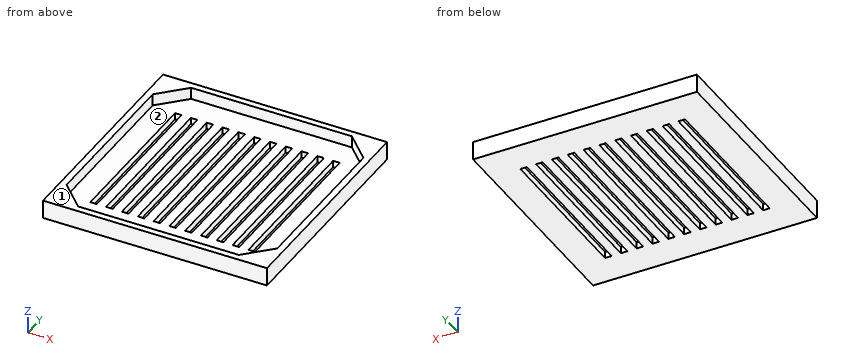
```python
from build123d import *

# Parameters (mm, degrees)
F0_W     = 85
F0_H     = 85
F1_DEPTH = 7
F3_DEPTH = 4.5
F4_W     = 2.5
F4_H     = 60
F5_DEPTH = 25


with BuildPart() as f1:
    # F0 (on Top) → F1 (new body)
    with BuildSketch(Plane.XY):
        Rectangle(F0_W, F0_H)
    extrude(amount=F1_DEPTH)

    # F2 (on face) → F3 (cut)
    with BuildSketch(Plane.XY.offset(7)):
        Polygon((30.5, 40), (-30.5, 40), (-40, 30.5), (-40, -30.5), (-30.5, -40), (30.5, -40), (40, -30.5), (40, 30.5), align=None)
    extrude(amount=-F3_DEPTH, mode=Mode.SUBTRACT)

    # F4 (on face) → F5 (cut)
    with BuildSketch(Plane.XY.offset(7)):
        with Locations((-30.000278, 0)):
            Rectangle(F4_W, F4_H)
        with Locations((-24.000278, 0)):
            Rectangle(F4_W, F4_H)
        with Locations((-18.000278, 0)):
            Rectangle(F4_W, F4_H)
        with Locations((-12.000278, 0)):
            Rectangle(F4_W, F4_H)
        with Locations((-6.000278, 0)):
            Rectangle(F4_W, F4_H)
        with Locations((-0.000278, 0)):
            Rectangle(F4_W, F4_H)
        with Locations((5.999722, 0)):
            Rectangle(F4_W, F4_H)
        with Locations((11.999722, 0)):
            Rectangle(F4_W, F4_H)
        with Locations((17.999722, 0)):
            Rectangle(F4_W, F4_H)
        with Locations((23.999722, 0)):
            Rectangle(F4_W, F4_H)
        with Locations((29.999722, 0)):
            Rectangle(F4_W, F4_H)
    extrude(amount=-F5_DEPTH, mode=Mode.SUBTRACT)


solid = f1.part
```
Design review of the part built by this model. Coordinates are the model's own, in mm. Face numbers are marked on the shaded views. Round coordinates to 2 decimals unless told otherwise and drop trailing zeros. Write each loop counter-clockwise with the first axis right and the second up, starting at its lowest first coordinate (ties: lowest second). Pieces come first, ordered by that corner, then holes. Notation, with made-up numbers: (29.25, 1) -> (72.25, 1) arc R25 ccw to (72.25, 29) -> close; hole circle Ø4 at (84.5, 37.25). An arc over 180 degrees is marked (long way). Answer in a Markdown table with one row per item.
Q1. Draft analysis for pull direction X (two halves, no side actions). For the marked faces 1 and 2, state which applies: +X half, -X half, draft (parallel to the pull), parting line (faces both ways), or undercut.
The answers:
| item | result |
|---|---|
| face 1 | draft |
| face 2 | undercut |
Q2. Take a section at C-C, the plane x = -27. State the section outline as (y, z) points, then the cut area to 3 significant figures.
The answers:
| item | result |
|---|---|
| outline | (-42.5, 0) -> (42.5, 0) -> (42.5, 7) -> (40, 7) -> (40, 2.5) -> (-40, 2.5) -> (-40, 7) -> (-42.5, 7) -> close |
| area | 235 mm² |
Q3. To check wall thickness, follow L1, parallel to X at y = -9.5, z = 5.25; L2, parallel to Z at x = -8, y = 23. State the ranges of each line that lie inside material, in increasing order. Write a range as [from, to].
The answers:
| item | result |
|---|---|
| L1 | [-42.5, -40], [40, 42.5] |
| L2 | [0, 2.5] |
Q4. Take a section at D-D, the plane z = 1.25. Count the separate pieces of the cut face and the enclosed holes in it, then the cut area to 4 significant figures.
The answers:
| item | result |
|---|---|
| separate pieces | 1 |
| enclosed holes | 11 |
| area | 5,575 mm² |
Q5. Take a section at B-B, the plane y = 33.5. State the section outline as (x, z) points.
The answers:
| item | result |
|---|---|
| outline | (-42.5, 0) -> (42.5, 0) -> (42.5, 7) -> (37, 7) -> (37, 2.5) -> (-37, 2.5) -> (-37, 7) -> (-42.5, 7) -> close |
Q6. Clearance check with flat-ended pins moving along their axes: pin 1 Ø6 at (x, y) = (32.5, 29.5) entering from +Z; pin 2 Ø5 at (x, y) = (-6, -21.5) entering from -Z. State where each tip first meets the part, or that it passes through.
The answers:
| item | result |
|---|---|
| pin 1 | z = 2.5 |
| pin 2 | z = 0 |
Q7. Take a section at A-A, the plane z = 6. State the section outline as (x, y) points, then the cut area to 3 significant figures.
The answers:
| item | result |
|---|---|
| outline | (-42.5, -42.5) -> (42.5, -42.5) -> (42.5, 42.5) -> (-42.5, 42.5) -> close; hole (-40, -30.5) -> (-30.5, -40) -> (30.5, -40) -> (40, -30.5) -> (40, 30.5) -> (30.5, 40) -> (-30.5, 40) -> (-40, 30.5) -> close |
| area | 1,010 mm² |
